Study the drawing (mm; zero at the part's minimum x, y, z) and answer. Round coordinates to 2 decimals unless told otherwise and drop trailing zeros. Loops run counter-clockwise (first coordinate to the right, second up) from the corner with the lowest first, then second, coordinate; pieces in that order, holes last. Notation, with made-up numbers: (7.5, 52.5) -> (55.5, 52.5) arc R20 cw to (55.5, 89.5) -> close; hole circle Ø10 at (39, 44.5). An arc over 180 degrees is marked (long way). Answer in a Markdown table with one row per item. Add a question column.
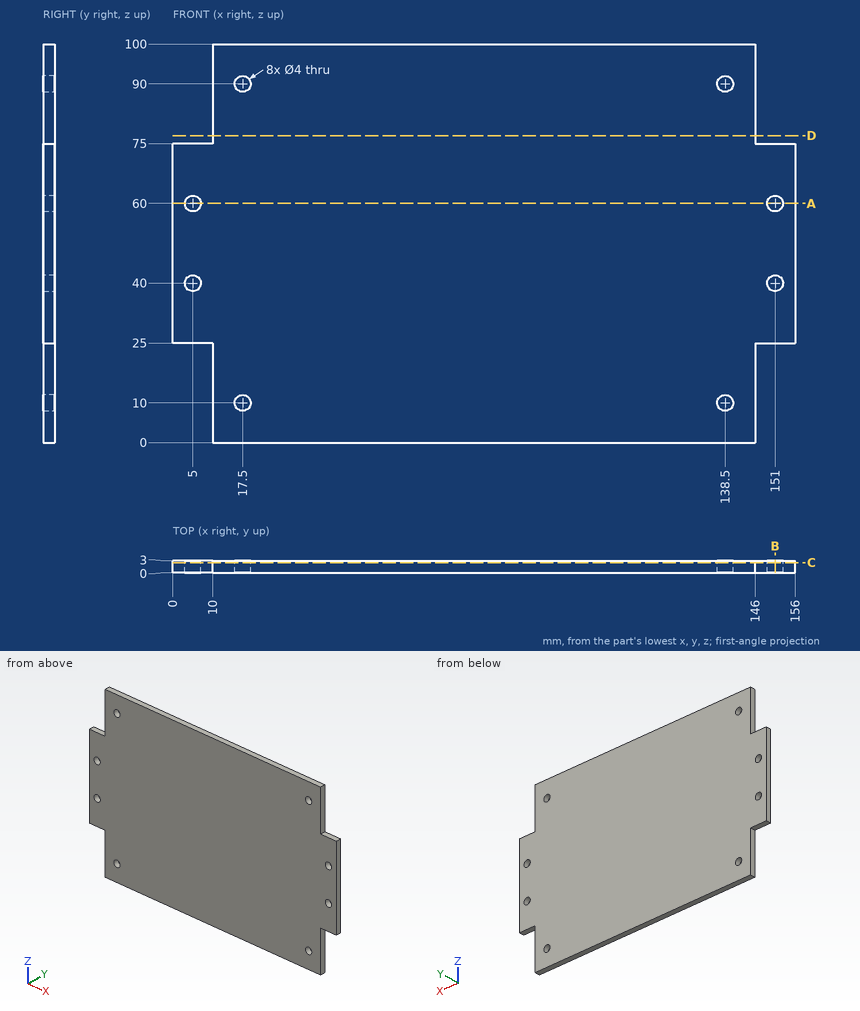
Item 1: Section D-D, the plane z = 77 is taken. Write down the section's boundary in (x, y).
Item 2: Flat-ended cylindrical pins translate along their axes: P1, Ø8, axis at x = 16.5, z = 13.5, coming from the -Y side; P2, Ø3.5, axis at x = 151, z = 60, coming from the +Y side; P3, Ø0.9, axis at x = 3, y = 2, coming from the +Z side; P4, Ø1.5, axis at y = 1.5, z = 83.5, coming from the -X side. Find the tip coordinate at first contact, or state that the pin passes through.
Item 3: Section A-A, the plane z = 60 is taken. Write down the section's boundary in (x, y).
Item 4: Section B-B, the plane x = 151 is taken. Write down the section's boundary in (y, z), and give its area (3 significant figures).
Item 5: Section C-C, the plane y = 2.5 is taken. Give the number of separate pieces and of enclosed holes in the cut face, and give its area (3 significant figures).
Item 6: Consider L1, parallel to Z at x = 17.5, y = 1.05; L2, parallel to Z at x = 151, y = 1; L3, parallel to X at y = 1.45, z = 40. Determine where each line is inside the solid, lowest interval first. Write a range as from..to.
Here are the results:
| question | item | result |
|---|---|---|
| 1 | outline | (10, 0) -> (146, 0) -> (146, 3) -> (10, 3) -> close |
| 2 | P1 | stops at y = 0 |
| 2 | P2 | passes through |
| 2 | P3 | stops at z = 75 |
| 2 | P4 | stops at x = 10 |
| 3 | outline | (0, 0) -> (3, 0) -> (3, 3) -> (0, 3) -> close; (7, 0) -> (149, 0) -> (149, 3) -> (7, 3) -> close; (153, 0) -> (156, 0) -> (156, 3) -> (153, 3) -> close |
| 4 | outline | (0, 25) -> (3, 25) -> (3, 38) -> (0, 38) -> close; (0, 42) -> (3, 42) -> (3, 58) -> (0, 58) -> close; (0, 62) -> (3, 62) -> (3, 75) -> (0, 75) -> close |
| 4 | area | 126 mm² |
| 5 | separate pieces | 1 |
| 5 | enclosed holes | 8 |
| 5 | area | 14,500 mm² |
| 6 | L1 | z = 0..8, 12..88, 92..100 |
| 6 | L2 | z = 25..38, 42..58, 62..75 |
| 6 | L3 | x = 0..3, 7..149, 153..156 |
